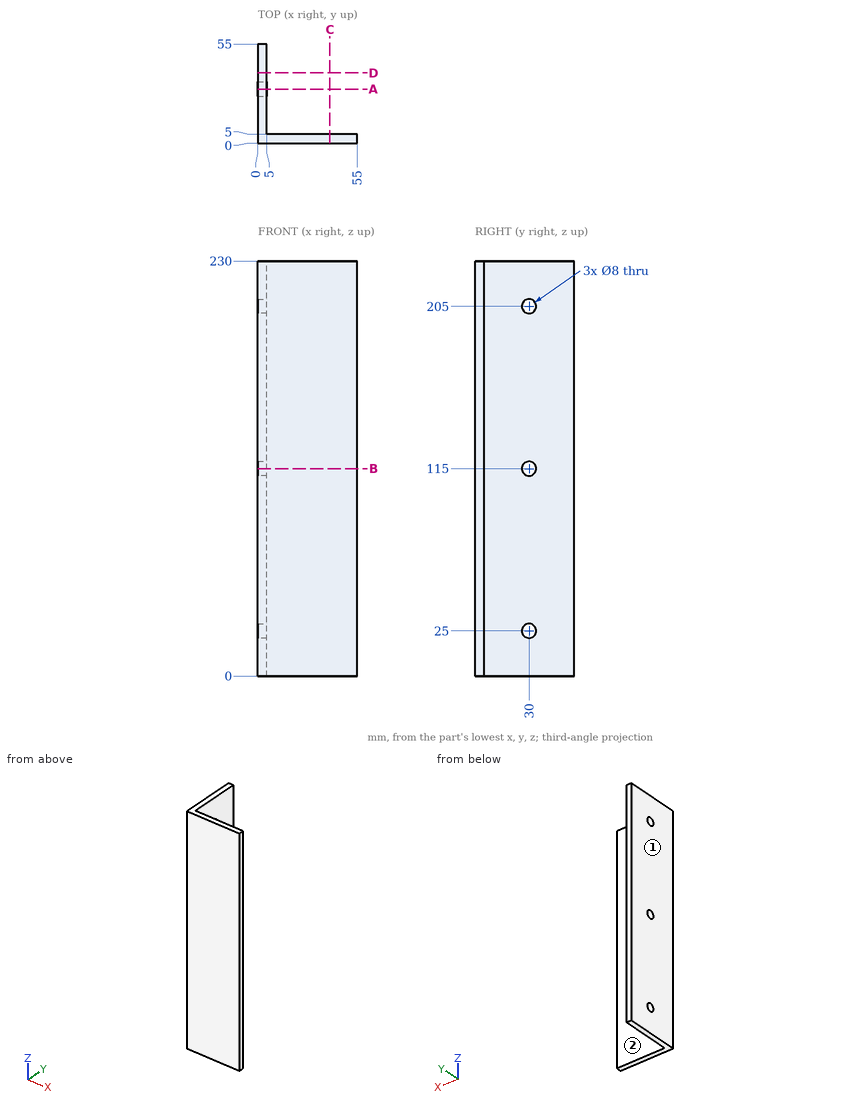
Study the drawing (mm; zero at the part's minimum x, y, z) and answer. A direction names the side the tool comes from. Coordinates: 2 decimals unless noted, no trailing zeros. Loops run counter-clockwise (first coordinate to the right, second up) from the corner with the lowest first, then second, coordinate; pieces in that order, holes last. Notation, with made-up numbers: M -12,19 L 4,19 A30 cw 4,41 Z; hole C 18.25,52 d10. An arc over 180 degrees is marked long. Answer in a Markdown table with one row per item.
1) Which of the six approach directions +Z, -Z, +X, -X, +Y, -Y give full straight-line access (tool end or side, diameter ignored) to the marked faces 1 and 2?
Answers below:
| item | result |
|---|---|
| face 1 | +Z, -Z, -X, +Y, -Y |
| face 2 | +Z, -Z, +X, +Y |
2) Find the intervals of material crossed by probe 1 along Y at (x, z) = (2, 115); probe 2 along Y at (x, z) = (45.5, 66), in increasing order.
Answers below:
| item | result |
|---|---|
| probe 1 | 0 to 26, 34 to 55 |
| probe 2 | 0 to 5 |
3) Find section A-A (y = 30). Determine the outline of the cut face in (x, z), then the cut area to 3 significant figures.
Answers below:
| item | result |
|---|---|
| outline | M 0,0 L 5,0 L 5,21 L 0,21 Z; M 0,29 L 5,29 L 5,111 L 0,111 Z; M 0,119 L 5,119 L 5,201 L 0,201 Z; M 0,209 L 5,209 L 5,230 L 0,230 Z |
| area | 1,030 mm^2 |
4) Find section C-C (x = 40). Determine the outline of the cut face in (y, z).
Answers below:
| item | result |
|---|---|
| outline | M 0,0 L 5,0 L 5,230 L 0,230 Z |
5) Given pin 1 (5 mm diameter, centred on y = 30, z = 115, fed in from -X); pin 2 (9 mm diameter, centred on y = 30, z = 25, fed in from +X), each flat-ended and moving along its own axis, determine where each tip first touches the part or whether it passes through.
Answers below:
| item | result |
|---|---|
| pin 1 | through |
| pin 2 | x = 5 |
6) Find section B-B (z = 115). Determine the outline of the cut face in (x, y).
Answers below:
| item | result |
|---|---|
| outline | M 0,0 L 55,0 L 55,5 L 5,5 L 5,26 L 0,26 Z; M 0,34 L 5,34 L 5,55 L 0,55 Z |
